Model file for the job. Use its own axes, mm. A direction names the side the tool comes from. Coordinates: 2 decimals unless noted, no trailing zeros. Write each loop counter-clockwise with the first axis right and the second up, starting at its lowest first coordinate (ties: lowest second). Pieces come first, ordered by that corner, then holes.
Q1. Which spindle directions (+Z, -Z, +X, -X, +Y, -Y) get a long thin tool onto all of the face, cutting with end or side? Do faces 1 (the flat face through (23, 5, 2)), 2 (the flat face through (69, 7, 5)). Say none if no direction does.
Q2. Band-saw the part on B-B, the plane x = 70. Write the cut outline in (y, z).
Q3. Band-saw the part on C-C, the plane z = 3.75. Write the cut outline in (x, y).
Q4. Drill centre lines: probe 1 along X at (y, z) = (5.25, 0.55); probe 2 along Y at (x, z) = (70, 3.55); probe 3 along Y at (x, z) = (129, 0.85). Where is each one in solid material? Low to high.
Q5. Band-saw the part on A-A, the plane y = 5. Write the cut outline in (x, z).
Q6. Pull direction Y, two halves, no side cores. Call faces 3 (the flat face through (69, 10, 2)), 4 (the flat face through (140, 5, 2)), 5 (the flat face through (137, 5, 2)): released by +Y, released by -Y, zero draft, split by the parting line, or undercut.
from build123d import *

# Parameters (mm, degrees)
F0_W     = 140
F0_H     = 10
F0_W_2   = 20
F0_H_2   = 3
F0_R     = 1.5
F1_DEPTH = 5


with BuildPart() as f1:
    # F0 (on Top) → F1 (new body)
    with BuildSketch(Plane.XY):
        with Locations((70, 5)):
            Rectangle(F0_W, F0_H)
        with Locations((13, 4.8)):
            Rectangle(F0_W_2, F0_H_2, mode=Mode.SUBTRACT)
        with Locations((127, 4.8)):
            Rectangle(F0_W_2, F0_H_2, mode=Mode.SUBTRACT)
        with Locations((70, 5)):
            Circle(F0_R, mode=Mode.SUBTRACT)
    extrude(amount=F1_DEPTH)


solid = f1.part
Answer sheet:
1. face 1: +Z, -Z
1. face 2: +Z, +X, -X, +Y, -Y
2. outline: (0, 0) - (3.5, 0) - (3.5, 5) - (0, 5) - close; (6.5, 0) - (10, 0) - (10, 5) - (6.5, 5) - close
3. outline: (0, 0) - (140, 0) - (140, 10) - (0, 10) - close; hole (3, 3.3) - (23, 3.3) - (23, 6.3) - (3, 6.3) - close; hole circle Ø3 at (70, 5); hole (117, 3.3) - (137, 3.3) - (137, 6.3) - (117, 6.3) - close
4. probe 1: x = 0 to 3, 23 to 68.52, 71.48 to 117, 137 to 140
4. probe 2: y = 0 to 3.5, 6.5 to 10
4. probe 3: y = 0 to 3.3, 6.3 to 10
5. outline: (0, 0) - (3, 0) - (3, 5) - (0, 5) - close; (23, 0) - (68.5, 0) - (68.5, 5) - (23, 5) - close; (71.5, 0) - (117, 0) - (117, 5) - (71.5, 5) - close; (137, 0) - (140, 0) - (140, 5) - (137, 5) - close
6. face 3: released by +Y
6. face 4: zero draft
6. face 5: undercut
